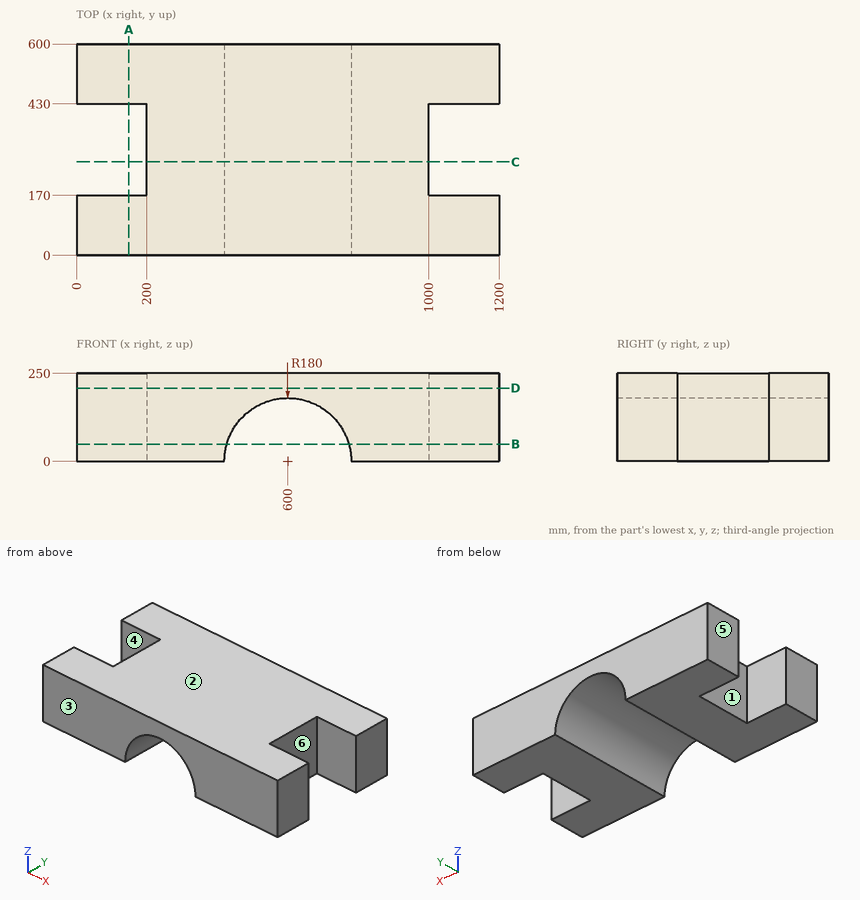
The drawing under review shows one solid part. Ordinate dimensions are in mm from its lowest x, y, z. A direction names the side the tool comes from. Coordinates: 2 decimals unless noted, no trailing zeros. Write each loop counter-clockwise with the first axis right and the second up, starting at its lowest first coordinate (ties: lowest second). Pieces come first, ordered by that corner, then holes.
1) Add section A-A (x = 149). Write out the cut boundary in (y, z), plus the area to 3 significant figures.
2) To check wall thickness, follow L1, parallel to Y at x = 173, z = 73.5; L2, parallel to X at y = 373, z = 59; L3, parallel to X at y = 570, z = 167. State the ranges of each line that lie inside material, in increasing order.
3) Add section D-D (z = 208). Write out the cut boundary in (x, y), plus the area to 3 significant figures.
4) Mouldability with a two-part tool opening along Y and no side actions: class the marked faces 1, 2 and 3 as +Y half, -Y half, draft (parallel to the pull), parting line (faces both ways), or undercut.
5) Add section B-B (z = 49). Write out the cut boundary in (x, y), plus the area to 3 significant figures.
6) Add section C-C (y = 265.5). Write out the cut boundary in (x, z).
7) Machinability: for the marked faces 4, 5 and 6, which of the approach directions +Z, -Z, +X, -X, +Y, -Y give a long, thin tool a straight path to every point of the face, cutting with its end or side? Answer none if there is none.
8) Insertion check: pin 1 (1.5 mm diameter, centred on y = 267, z = 135.5, fed in from +X); pin 2 (8 mm diameter, centred on y = 207, z = 212.5, fed in from -X). Each pin has a flat end and moves straight along its axis. Give the tip position at first contact, or say it passes through.
Check result:
1. outline: (0, 0) - (170, 0) - (170, 250) - (0, 250) - close; (430, 0) - (600, 0) - (600, 250) - (430, 250) - close
1. area: 85,000 mm2
2. L1: y = 0 to 170, 430 to 600
2. L2: x = 200 to 429.94, 770.06 to 1000
2. L3: x = 0 to 532.84, 667.16 to 1200
3. outline: (0, 0) - (1200, 0) - (1200, 170) - (1000, 170) - (1000, 430) - (1200, 430) - (1200, 600) - (0, 600) - (0, 430) - (200, 430) - (200, 170) - (0, 170) - close
3. area: 616,000 mm2
4. face 1: undercut
4. face 2: draft
4. face 3: -Y half
5. outline: (0, 0) - (426.8, 0) - (426.8, 600) - (0, 600) - (0, 430) - (200, 430) - (200, 170) - (0, 170) - close; (773.2, 0) - (1200, 0) - (1200, 170) - (1000, 170) - (1000, 430) - (1200, 430) - (1200, 600) - (773.2, 600) - close
5. area: 408,000 mm2
6. outline: (200, 0) - (420, 0) arc R180 cw to (780, 0) - (1000, 0) - (1000, 250) - (200, 250) - close
7. face 4: +Z, -Z, -X
7. face 5: +Z, -Z, -X, +Y, -Y
7. face 6: +Z, -Z, +X
8. pin 1: stops at x = 1000
8. pin 2: stops at x = 200
